Answer from the drawing. Dimensions are ordinates in mm from the lowest x, y and z of the part. A direction names the side the tool comes from. Give positions to 0.01 mm unless a question says otherwise; leave off trailing zeros. Order: outer loops, then holes, each group sorted by start corner. A loop starts at its lowest first (then second) coordinate and runs counter-clockwise, first axis right, second up. Notation, with made-up numbers: (49.25, -25.5) -> (102.25, -25.5) arc R30 cw to (102.25, -3.5) -> close; hole circle Ø4 at (25, 88). An arc over 180 degrees is marked (long way). Write item = value, one per line. Start each with the question number.
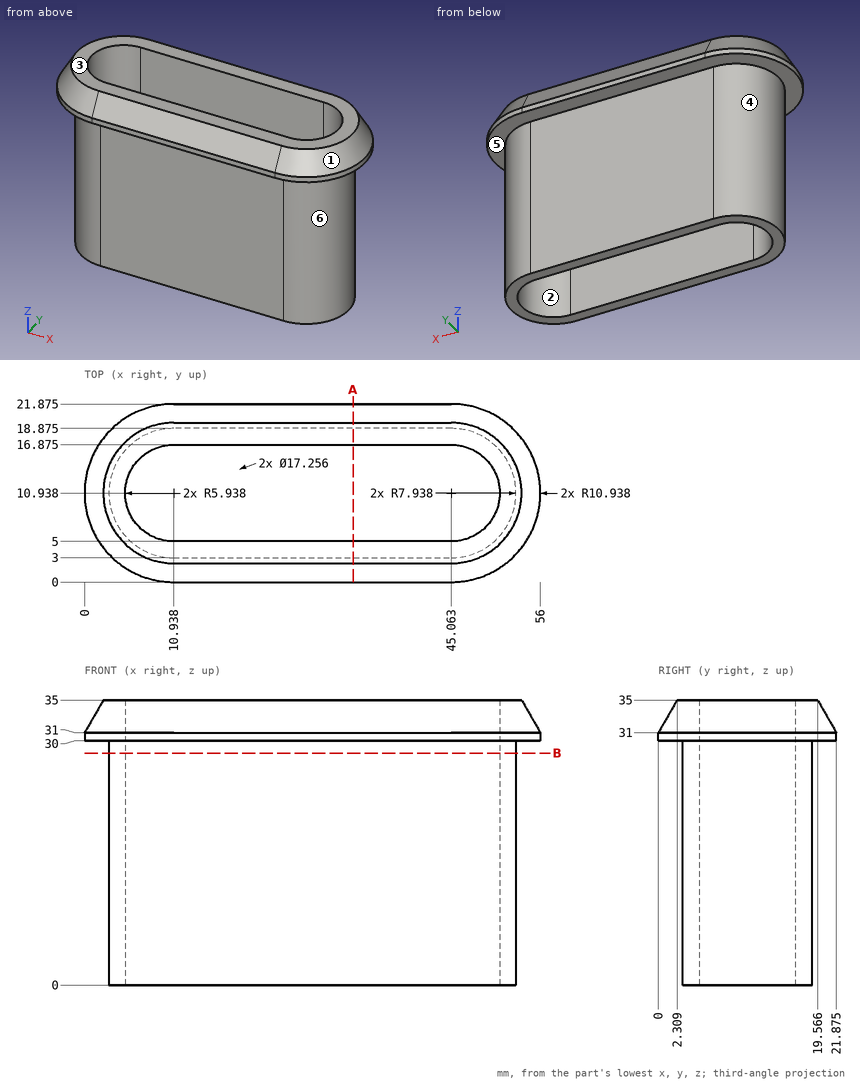
Item 1: Consider L1, parallel to Y at x = 32.5, z = 25 (1 decimal); L2, parallel to Z at x = 45, y = 19.25; L3, parallel to X at y = 12.25, z = 8. Determine where each line is inside the solid, lowest interval first. Write a range as from..to.
Item 2: The mould has two halves that part along Y. Classify the marked faces 1, 2 and 3: +Y half, -Y half, draft (parallel to the pull), parting line (faces both ways), or undercut.
Item 3: A cutting plane is placed at B-B, the plane z = 28.5. Write down the section's boundary in (x, y) (1 decimal).
Item 4: A cutting plane is placed at A-A, the plane x = 33. Write down the section's boundary in (y, z) (1 decimal).
Item 5: Which of the six approach directions +Z, -Z, +X, -X, +Y, -Y give full straight-line access (tool end or side, diameter ignored) to the marked faces 4, 5 and 6?
Item 6: Flat-ended cylindrical pins translate along their axes: pin 1 (9 mm diameter, centred on x = 31, z = 20, fed in from -Y); pin 2 (2 mm diameter, centred on x = 26.5, z = 26.5, fed in from +Y) (1 decimal); pin 3 (8 mm diameter, centred on y = 10, z = 4, fed in from +X). Find the tip coordinate at first contact, or state that the pin passes through.
Check values:
q1.L1 = 3..5, 16.9..18.9
q1.L2 = 30..35
q1.L3 = 3.11..5.15, 50.85..52.89
q2.face_1 = parting line
q2.face_2 = undercut
q2.face_3 = draft
q3.outline = (10.9, 3) -> (45.1, 3) arc R7.9 ccw to (45.1, 18.9) -> (10.9, 18.9) arc R7.9 ccw to start; hole (10.9, 5) -> (45.1, 5) arc R5.9 ccw to (45.1, 16.9) -> (10.9, 16.9) arc R5.9 ccw to start
q4.outline = (0, 30) -> (3, 30) -> (3, 0) -> (5, 0) -> (5, 35) -> (2.3, 35) -> (0, 31) -> close; (16.9, 0) -> (18.9, 0) -> (18.9, 30) -> (21.9, 30) -> (21.9, 31) -> (19.6, 35) -> (16.9, 35) -> close
q5.face_4 = -Z, -X
q5.face_5 = -Z
q5.face_6 = -Z, +X
q6.pin_1 = 3
q6.pin_2 = 18.9
q6.pin_3 = 53
